Here's how the part is built. I have some questions about the finished solid (model axes, mm). A direction names the side the tool comes from. Round coordinates to 2 decimals unless told otherwise and drop trailing zeros. Order: outer loops, then holes, each group sorted by start corner. A loop starts at its lowest first (then second) coordinate and runs counter-clockwise, first axis right, second up. Notation, with made-up numbers: M 2.25,14 L 13.25,14 A10 cw 13.25,22 Z; hole C 51,-4 d2. An arc over 180 degrees is marked long. Write item = value, one per line. Start each with the question number.
Item 1: I want a section at C-C, the plane x = 4. List the corners of the cut face in (y, z) for me.
Item 2: We'd pull the mould along Z, two halves only. Please class faces 1 (the face through (25, -3, 11)), 2 (the face through (19.08, -2.38, -10.74)), 3 (the face through (12.675, 7.91, -10.316)): pulls with the +Z half, pulls with the -Z half, needs draft (parallel to the pull), parting line crosses it, or undercut.
Item 3: I want a section at D-D, the plane x = 15.25. List the corners of the cut face in (y, z) for me, plus the area to 3 significant figures.
Item 4: Please list where these lines run through material, in increasing order: L1, parallel to Z at x = 21, y = 0; L2, parallel to Z at x = 6, y = 0; L3, parallel to X at y = -8.5, z = -5.5.
Item 5: I want a section at A-A, the plane y = 0. List the corners of the cut face in (x, z) for me, plus the area to 3 significant figures.
Item 6: I'm going to push flat-ended pins straight in: P1, Ø1.5, axis at y = 0, z = 8.5, coming from the +X side; P2, Ø11, axis at y = 3, z = 3.5, coming from the +X side; P3, Ø4, axis at x = 22.5, y = 10, coming from the -Z side; P4, Ø1.5, axis at x = 21, z = -2, coming from the +Y side. Where does each tip first touch, or does it pass through?
Item 7: For faces 4 (the face through (13, -10, 0)), 5 (the face through (0, 10, -1)), which set-ups out of +Z, -Z, +X, -X, +Y, -Y let a thin tool reach every point of the face, with its end or its side?
```python
from build123d import *

# Parameters (mm, degrees)
F0_W     = 25
F0_H     = 13
F2_R     = 9.5
F3_DEPTH = 57.5
F2_R_2   = 11
F4_DEPTH = 12


with BuildPart() as f1:
    # F0 (on Front) → F1 (revolve)
    with BuildSketch(Plane.XZ):
        with Locations((12.5, 6.5)):
            Rectangle(F0_W, F0_H)
    revolve(axis=Axis((12.5, 0, 0), (1, 0, 0)))

    # F2 (on face) → F3 (cut)
    with BuildSketch(Plane.YZ.offset(25)):
        Circle(F2_R)
    extrude(amount=-F3_DEPTH, mode=Mode.SUBTRACT)

    # F2 (on face) → F4 (cut)
    with BuildSketch(Plane.YZ.offset(25)):
        Circle(F2_R_2)
        Circle(F2_R, mode=Mode.SUBTRACT)
    extrude(amount=-F4_DEPTH, mode=Mode.SUBTRACT)


solid = f1.part
```
Filled in:
q1.outline = C 0,0 d26; hole C 0,0 d19
q2.face_1 = needs draft
q2.face_2 = undercut
q2.face_3 = parting line crosses it
q3.outline = C 0,0 d26; hole C 0,0 d22
q3.area = 151 mm^2
q4.L1 = -13 to -11, 11 to 13
q4.L2 = -13 to -9.5, 9.5 to 13
q4.L3 = 0 to 13
q5.outline = M 0,-13 L 25,-13 L 25,-11 L 13,-11 L 13,-9.5 L 0,-9.5 Z; M 0,9.5 L 13,9.5 L 13,11 L 25,11 L 25,13 L 0,13 Z
q5.area = 139 mm^2
q6.P1 = through
q6.P2 = 13
q6.P3 = -10.25
q6.P4 = 12.94
q7.face_4 = +X
q7.face_5 = +Z, -Z, -X, +Y, -Y
